The listing builds one solid part. Answer for the finished solid, in the listing's coordinates (mm). Give positions to 0.01 mm unless a question says otherwise; leave off trailing zeros. Order: outer loops, then holes, each group sorted by start corner. A loop starts at its lowest first (then second) coordinate and runs counter-clockwise, first axis right, second up. Notation, with made-up numbers: (68.25, 77) - (114.25, 77) arc R20 ccw to (114.25, 84) - close; hole circle Ø11 at (28.25, -2.5). An arc over 180 degrees is marked (long way). Use CSV: the item, a comma, the result in double quotes.
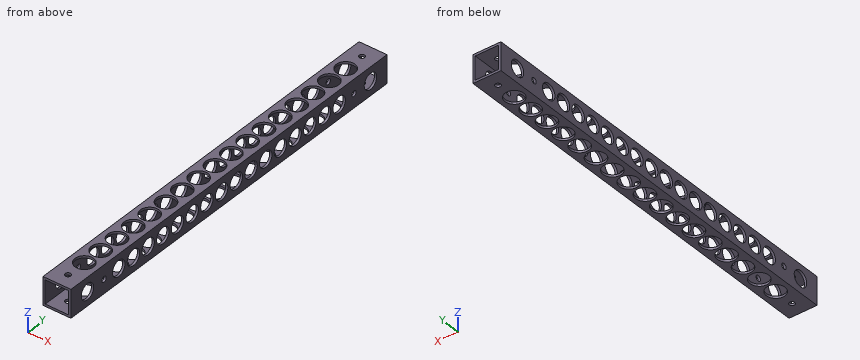
Autodesk Inventor part; units mm, degrees
ref_plane "YZ Plane" through (0, 0, 0) normal (1, 0, 0) x (0, 1, 0)
ref_plane "XZ Plane" through (0, 0, 0) normal (0, 1, 0) x (-1, 0, 0)
ref_plane "XY Plane" through (0, 0, 0) normal (0, 0, 1) x (1, 0, 0)
sketch "スケッチ1" plane through (0, 0, 0) normal (0, 1, 0) x (-1, 0, 0)
  line L0 (0, 0) -> (-15, 0)
  line L1 (-15, 0) -> (-15, 15)
  line L2 (-15, 15) -> (0, 15)
  line L3 (0, 15) -> (0, 0)
  line L4 (-1.2, 13.8) -> (-13.8, 13.8)
  line L5 (-13.8, 13.8) -> (-13.8, 1.2)
  line L6 (-13.8, 1.2) -> (-1.2, 1.2)
  line L7 (-1.2, 1.2) -> (-1.2, 13.8)
  dimension "d0" = 15
  dimension "d1" = 15
  dimension "d2" = 1.2
  dimension "d3" = 1.2
  dimension "d4" = 1.2
  dimension "d5" = 1.2
extrude "押し出し1" add sketch "スケッチ1" along normal blind 215
sketch "スケッチ2" plane through (0, 0, 15) normal (0, 0, 1) x (1, 0, 0)
  line L0 (0, 0) -> (0, 215)
  line L1 (0, 0) -> (15, 0)
  line L2 (0, 215) -> (15, 215)
  point P0 (7.5, 7.5)
  point P1 (7.5, 207.5)
  dimension "d8" = 7.5
  dimension "d9" = 7.5
  dimension "d10" = 7.5
  dimension "d11" = 7.5
hole "穴1" at (7.5, 7.5, 15) at (7.5, 207.5, 15) direction (0, 0, -1) diameter 3 end through all
sketch "スケッチ3" plane through (0, 0, 0) normal (-1, 0, 0) x (0, 0, 1)
  line L0 (0, 0) -> (0, 215)
  line L1 (0, 0) -> (15, 0)
  line L2 (0, 215) -> (15, 215)
  point P0 (7.5, 22.5)
  point P1 (7.5, 192.5)
  dimension "d19" = 7.5
  dimension "d20" = 7.5
  dimension "d21" = 22.5
  dimension "d22" = 22.5
hole "穴2" at (0, 22.5, 7.5) at (0, 192.5, 7.5) direction (1, 0, 0) diameter 3 end through all
sketch "スケッチ4" plane through (15, 0, 15) normal (1, 0, 0) x (0, 0, -1)
  line L0 (0, 0) -> (15, 0)
  circle A0 centre (7.5, 22.5) radius 1.5
  line L1 (15, 0) -> (15, 215)
  line L2 (0, 215) -> (15, 215)
  circle A1 centre (7.5, 192.5) radius 1.5
  point P0 (7.5, 11.25)
  point P1 (7.5, 203.75)
  point P2 (7.5, 182.5)
  point P3 (7.5, 172.5)
  point P4 (7.5, 162.5)
  point P5 (7.5, 152.5)
  point P6 (7.5, 142.5)
  point P7 (7.5, 132.5)
  point P8 (7.5, 122.5)
  point P9 (7.5, 112.5)
  point P10 (7.5, 102.5)
  point P11 (7.5, 92.5)
  point P12 (7.5, 82.5)
  point P13 (7.5, 72.5)
  point P14 (7.5, 62.5)
  point P15 (7.5, 52.5)
  point P16 (7.5, 42.5)
  point P17 (7.5, 32.5)
  dimension "d30" = 22.5
  dimension "d31" = 11.25
  dimension "d32" = 7.5
  dimension "d33" = 11.25
  dimension "d34" = 7.5
  dimension "d35" = 170
  dimension "d36" = 7.5
  dimension "d37" = 10
  dimension "d40" = 10
hole "穴3" at (15, 11.25, 7.5) at (15, 203.75, 7.5) at (15, 182.5, 7.5) at (15, 172.5, 7.5) at (15, 162.5, 7.5) at (15, 152.5, 7.5) at (15, 142.5, 7.5) at (15, 132.5, 7.5) at (15, 122.5, 7.5) at (15, 112.5, 7.5) at (15, 102.5, 7.5) at (15, 92.5, 7.5) at (15, 82.5, 7.5) at (15, 72.5, 7.5) at (15, 62.5, 7.5) at (15, 52.5, 7.5) at (15, 42.5, 7.5) at (15, 32.5, 7.5) direction (-1, 0, 0) diameter 8.5 end through all
sketch "スケッチ5" plane through (0, 0, 15) normal (0, 0, 1) x (1, 0, 0)
  circle A0 centre (7.5, 7.5) radius 1.5
  circle A1 centre (7.5, 207.5) radius 1.5
  line L0 (15, 0) -> (15, 215)
  point P0 (0, 0)
  point P1 (7.5, 196.3889)
  point P2 (7.5, 185.2778)
  point P3 (7.5, 174.1667)
  point P4 (7.5, 163.0556)
  point P5 (7.5, 151.9444)
  point P6 (7.5, 140.8333)
  point P7 (7.5, 129.7222)
  point P8 (7.5, 118.6111)
  point P9 (7.5, 107.5)
  point P10 (7.5, 96.3889)
  point P11 (7.5, 85.2778)
  point P12 (7.5, 74.1667)
  point P13 (7.5, 63.0556)
  point P14 (7.5, 51.9444)
  point P15 (7.5, 40.8333)
  point P16 (7.5, 29.7222)
  point P17 (7.5, 18.6111)
  dimension "d52" = 200
  dimension "d53" = 7.5
  dimension "d56" = 11.1111
  dimension "d61" = 11.1111
hole "穴4" at (7.5, 196.3889, 15) at (7.5, 185.2778, 15) at (7.5, 174.1667, 15) at (7.5, 163.0556, 15) at (7.5, 151.9444, 15) at (7.5, 140.8333, 15) at (7.5, 129.7222, 15) at (7.5, 118.6111, 15) at (7.5, 107.5, 15) at (7.5, 96.3889, 15) at (7.5, 85.2778, 15) at (7.5, 74.1667, 15) at (7.5, 63.0556, 15) at (7.5, 51.9444, 15) at (7.5, 40.8333, 15) at (7.5, 29.7222, 15) at (7.5, 18.6111, 15) direction (0, 0, -1) diameter 10 end through all
equation "\"d3\" = d2"
equation "\"d4\" = d3"
equation "\"d5\" = d2"
properties part number "ロボットベース15x15_2" material "アルミニウム 6061"
Item 1: Find the intervals of material crossed by line 1 along Z through (x, y) = (0.65, 11.25); line 2 along X through (y, z) = (109, 4.75), in increasing order.
Taken from the geometry:
line 1,"0 to 3.25, 11.75 to 15"
line 2,"0 to 1.2, 13.8 to 15"
Item 2: The part is cut by section A-A (y = 203.75). Give the vertices of the cut face in (x, z).
Taken from the geometry:
outline,"(0, 0) - (15, 0) - (15, 3.25) - (13.8, 3.25) - (13.8, 1.2) - (1.2, 1.2) - (1.2, 3.25) - (0, 3.25) - close; (0, 11.75) - (1.2, 11.75) - (1.2, 13.8) - (13.8, 13.8) - (13.8, 11.75) - (15, 11.75) - (15, 15) - (0, 15) - close"
Item 3: The part is cut by section D-D (y = 50.5). Give the vertices of the cut face in (x, z), and give its area (3 significant figures).
Taken from the geometry:
outline,"(0, 0) - (2.71, 0) - (2.71, 1.2) - (1.2, 1.2) - (1.2, 3.75) - (0, 3.75) - close; (0, 11.25) - (1.2, 11.25) - (1.2, 13.8) - (2.71, 13.8) - (2.71, 15) - (0, 15) - close; (12.29, 0) - (15, 0) - (15, 3.75) - (13.8, 3.75) - (13.8, 1.2) - (12.29, 1.2) - close; (12.29, 13.8) - (13.8, 13.8) - (13.8, 11.25) - (15, 11.25) - (15, 15) - (12.29, 15) - close"
area,"25.3 mm^2"
Item 4: This flat-tipped pin is pushed along its axis until it touches: pin 1 (1 mm diameter, centred on x = 11.5, z = 6, fed in from +Y). Where does it stop, or does it pass through?
Taken from the geometry:
pin 1,"through"
Item 5: The part is cut by section B-B (y = 142.5). Give the vertices of the cut face in (x, z), and give its area (3 significant figures).
Taken from the geometry:
outline,"(0, 0) - (2.79, 0) - (2.79, 1.2) - (1.2, 1.2) - (1.2, 3.25) - (0, 3.25) - close; (0, 11.75) - (1.2, 11.75) - (1.2, 13.8) - (2.79, 13.8) - (2.79, 15) - (0, 15) - close; (12.21, 0) - (15, 0) - (15, 3.25) - (13.8, 3.25) - (13.8, 1.2) - (12.21, 1.2) - close; (12.21, 13.8) - (13.8, 13.8) - (13.8, 11.75) - (15, 11.75) - (15, 15) - (12.21, 15) - close"
area,"23.2 mm^2"
Item 6: The part is cut by section C-C (x = 10.75). Count the separate pieces of the cut face and the enclosed holes in it, and give its area (3 significant figures).
Taken from the geometry:
separate pieces,"36"
enclosed holes,"0"
area,"206 mm^2"
